from build123d import *

# Parameters (mm, degrees)
SKETCH1_W                = 50
SKETCH1_H                = 50
BOSS_EXTRUDE1_DEPTH      = 50
CHAMFER1_SIZE            = 10
CHAMFER2_SIZE            = 1.5
BOSS_EXTRUDE2_DEPTH      = 7
BOSS_EXTRUDE2_DEPTH_BACK = 10
SKETCH10_W               = 1
SKETCH10_H               = 7
SKETCH11_W               = 1.8
SKETCH11_H               = 1.8
CUT_EXTRUDE1_DEPTH       = 7


with BuildPart() as part:
    # Sketch1 → Boss-Extrude1 (new body)
    with BuildSketch(Plane.XY):
        with Locations((25, 25)):
            Rectangle(SKETCH1_W, SKETCH1_H)
    extrude(amount=BOSS_EXTRUDE1_DEPTH)

    # Cut-Sweep5: sweep along a path in Sketch9
    with BuildLine(Plane(origin=(0, 25, 0), x_dir=(-1, 0, 0), z_dir=(0, -1, 0))) as cut_sweep5_path:
        Line((-50, -25), (-39, -25))
        ThreePointArc((-39, -25), (-29.100505063, -29.100505063), (-25, -39))
        Line((-25, -39), (-25, -50))
    # Sketch8 → Cut-Sweep5 (sweep, cut)
    with BuildSketch(Plane(origin=(50, 0, 0), x_dir=(0, 0, -1), z_dir=(1, 0, 0))):
        Polygon((-14, 29.556349186), (-20.443650814, 36), (-29.556349186, 36), (-36, 29.556349186), (-36, 20.443650814), (-29.556349186, 14), (-20.443650814, 14), (-14, 20.443650814), align=None)
    sweep(path=cut_sweep5_path.line, mode=Mode.SUBTRACT)

    # Chamfer1
    chamfer1_edges = [part.edges().sort_by_distance(p)[0] for p in [
        (17.221825407, 17.221825407, 50),
        (32.778174593, 17.221825407, 50),
        (36, 25, 50),
        (32.778174593, 32.778174593, 50),
        (17.221825407, 32.778174593, 50),
        (14, 25, 50),
        (25, 14, 50),
        (25, 36, 50),
    ]]
    chamfer(chamfer1_edges, length=CHAMFER1_SIZE)

    # Chamfer2
    chamfer2_edges = [part.edges().sort_by_distance(p)[0] for p in [
        (50, 25, 50),
        (25, 50, 50),
        (0, 25, 50),
        (25, 50, 0),
        (50, 25, 0),
        (25, 0, 0),
        (0, 25, 0),
        (25, 0, 50),
        (0, 50, 25),
        (50, 50, 25),
        (50, 0, 25),
        (0, 0, 25),
    ]]
    chamfer(chamfer2_edges, length=CHAMFER2_SIZE)

    # Sketch10 → Boss-Extrude2 (add, two sides: drawn at the far end of the back side and taken through both)
    with BuildSketch(Plane.XY.offset(50).offset(-BOSS_EXTRUDE2_DEPTH_BACK)):
        with Locations((0.5, 25)):
            Rectangle(SKETCH10_W, SKETCH10_H)
    extrude(amount=BOSS_EXTRUDE2_DEPTH + BOSS_EXTRUDE2_DEPTH_BACK)

    # Sketch11 → Cut-Extrude1 (cut)
    with BuildSketch(Plane(origin=(1, 0, 0), x_dir=(0, 0, -1), z_dir=(1, 0, 0))):
        with Locations((-53.6, 25)):
            Rectangle(SKETCH11_W, SKETCH11_H)
    extrude(amount=-CUT_EXTRUDE1_DEPTH, mode=Mode.SUBTRACT)


solid = part.part
Input: part model. Units: mm. Frame: model coordinates. A direction names the side the tool comes from. Coordinates: 2 decimals unless noted, no trailing zeros. Order: outer loops, then holes, each group sorted by start corner. A loop starts at its lowest first (then second) coordinate and runs counter-clockwise, first axis right, second up. Notation, with made-up numbers: M 66,78 L 87,78 A13 cw 87,96 Z; hole C 60,74 d7. An arc over 180 degrees is marked long. Answer as CSV lines item,"result".
1. Section B-B (x = 45). Return the cut outline in (y, z), then the cut area to 3 significant figures.
Reported:
outline,"M 0,1.5 L 1.5,0 L 48.5,0 L 50,1.5 L 50,48.5 L 48.5,50 L 34.7,50 L 33.28,49 L 16.72,49 L 15.3,50 L 1.5,50 L 0,48.5 Z; hole M 14,20.44 L 20.44,14 L 29.56,14 L 36,20.44 L 36,29.56 L 29.56,36 L 20.44,36 L 14,29.56 Z"
area,"2,080 mm2"
2. Pull-direction query (Y, two-part tool) for faces 1 (the flat face through (0.8, 49.3, 24.7)), 2 (the cylindrical face through (36.9, 24.94, 36.86)), 3 (the flat face through (1, 1, 1)); classes: released by +Y, released by -Y, zero draft, split by the parting line, or undercut.
Reported:
face 1,"released by +Y"
face 2,"undercut"
face 3,"released by -Y"
3. First-contact query: P1, Ø5, axis at x = 26, y = 27.5, coming from the +Z side; P2, Ø3.5, axis at y = 24, z = 54.5, coming from the +X side; P3, Ø0.5, axis at x = 0.5, y = 24.5, coming from the -Z side. Flat tips, straight axial feed; report the tip coordinate or a pass-through.
Reported:
P1,"z = 19.38"
P2,"x = 1"
P3,"z = 0.75"
4. Section C-C (y = 6.5). Return the cut outline in (x, z).
Reported:
outline,"M 0,1.5 L 1.5,0 L 48.5,0 L 50,1.5 L 50,48.5 L 48.5,50 L 36.2,50 L 32.66,47.5 L 17.34,47.5 L 13.8,50 L 1.5,50 L 0,48.5 Z"
5. Section D-D (x = 5.5). Return the cut outline in (y, z).
Reported:
outline,"M 0,1.5 L 1.5,0 L 48.5,0 L 50,1.5 L 50,48.5 L 48.5,50 L 35.2,50 L 33.08,48.5 L 16.92,48.5 L 14.8,50 L 1.5,50 L 0,48.5 Z"
6. Section A-A (y = 31). Return the cut outline in (x, z), then the cut area to 3 significant figures.
Reported:
outline,"M 0,1.5 L 1.5,0 L 48.5,0 L 50,1.5 L 50,15.44 L 39,15.44 A23.56 cw 15.44,39 L 15.44,40 L 10.51,43.49 L 4,50 L 1.5,50 L 0,48.5 Z; M 34.56,39 A4.44 ccw 39,34.56 L 50,34.56 L 50,48.5 L 48.5,50 L 46,50 L 39.49,43.49 L 34.56,40 Z"
area,"1,530 mm2"
7. Material intervals for line 1 (Y direction, x = 30, z = 27.5); line 2 (X direction, y = 35, z = 49); line 3 (Y direction, x = 28.5, z = 48), sorted ascending. Write a range as from..to.
Reported:
line 1,"0..14, 36..50"
line 2,"0.5..6.72, 43.28..49.5"
line 3,"0..6, 44..50"
8. Access query for faces 4 (the flat face through (44.423, 32.733, 17.177)), 5 (the flat face through (35, 36, 28)), 6 (the flat face through (17.177, 32.733, 39.507)). Directions: +Z, -Z, +X, -X, +Y, -Y. A direction counts if a zero-diameter tool reaches every point of the face in a straight line with its end or side. Return the directions, or none.
Reported:
face 4,"+X"
face 5,"none"
face 6,"+Z"
